Print and shaded views of the part. All mm, measured from the part's lowest x, y and z. Give positions to 0.01 mm unless a question says otherwise; leave off trailing zeros. Loops run counter-clockwise (first coordinate to the right, second up) from the corner with the lowest first, then second, coordinate; pieces in that order, holes last. Notation, with made-up numbers: M -30,-1 L -13,-1 A6 ccw -13,10 Z; hole C 74,-18.5 d7. An arc over 180 degrees is marked long. Answer in a Markdown table with one row per item.
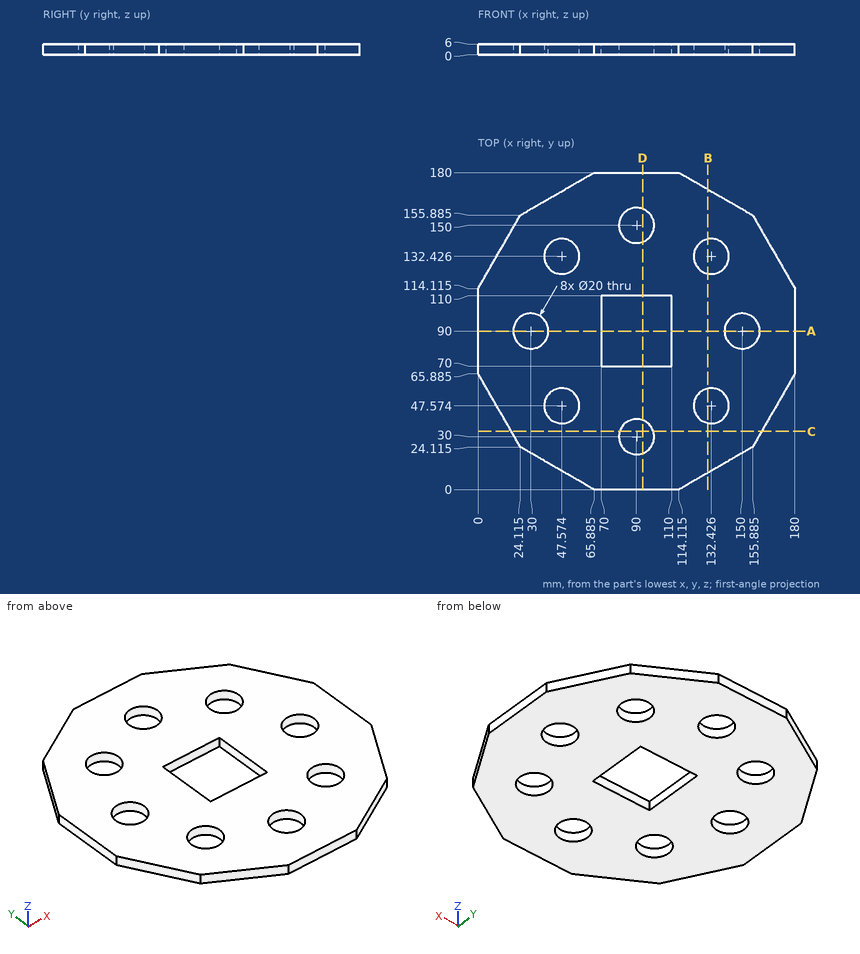
(1) Saw through at B-B, the plane x = 130.5. Give the cut face in (y, z).
Established:
| item | result |
|---|---|
| outline | M 9.46,0 L 37.76,0 L 37.76,6 L 9.46,6 Z; M 57.39,0 L 122.61,0 L 122.61,6 L 57.39,6 Z; M 142.24,0 L 170.54,0 L 170.54,6 L 142.24,6 Z |
(2) Flat gauge pins, fed straight in: P1, Ø2, axis at y = 39.5, z = 4, coming from the -X side (1 decimal); P2, Ø18, axis at x = 150, y = 90, coming from the +Z side; P3, Ø1.5, axis at x = 20.5, z = 4.5, coming from the +Y side; P4, Ø1.5, axis at x = 140, z = 5, coming from the +Y side. Where does each tip first touch, or does it go through?
Established:
| item | result |
|---|---|
| P1 | stops at x = 14.7 |
| P2 | passes through |
| P3 | stops at y = 150.92 |
| P4 | stops at y = 165.49 |
(3) Saw through at A-A, the plane y = 90. Give the cut face in (x, z).
Established:
| item | result |
|---|---|
| outline | M 0,0 L 20,0 L 20,6 L 0,6 Z; M 40,0 L 70,0 L 70,6 L 40,6 Z; M 110,0 L 140,0 L 140,6 L 110,6 Z; M 160,0 L 180,0 L 180,6 L 160,6 Z |
(4) Wall check: L1, parallel to X at y = 101, z = 3.1; L2, parallel to Y at x = 42, z = 4.25 (1 decimal); L3, parallel to Y at x = 50.5, z = 4.75 (1 decimal). Give the ranges that are in metal, low to high.
Established:
| item | result |
|---|---|
| L1 | x = 0 to 70, 110 to 180 |
| L2 | y = 13.8 to 39.3, 55.9 to 124.1, 140.7 to 166.2 |
| L3 | y = 8.9 to 38, 57.1 to 122.9, 142 to 171.1 |
(5) Saw through at C-C, the plane y = 33. Give the cut face in (x, z).
Established:
| item | result |
|---|---|
| outline | M 18.99,0 L 80.46,0 L 80.46,6 L 18.99,6 Z; M 99.54,0 L 161.01,0 L 161.01,6 L 99.54,6 Z |
(6) Saw through at D-D, the plane x = 93.5. Give the cut face in (y, z), and give its area (3 significant figures).
Established:
| item | result |
|---|---|
| outline | M 0,0 L 20.63,0 L 20.63,6 L 0,6 Z; M 39.37,0 L 70,0 L 70,6 L 39.37,6 Z; M 110,0 L 140.63,0 L 140.63,6 L 110,6 Z; M 159.37,0 L 180,0 L 180,6 L 159.37,6 Z |
| area | 615 mm2 |
